Design review of the part built by this model. Coordinates are the model's own, in mm. Face numbers are marked on the shaded views. Round coordinates to 2 decimals unless told otherwise and drop trailing zeros. Loops run counter-clockwise (first coordinate to the right, second up) from the corner with the lowest first, then second, coordinate; pieces in that order, holes last. Notation, with made-up numbers: M 24.5,-4.75 L 69.5,-4.75 A25 cw 69.5,30.25 Z; hole C 74.25,26 d11. An arc over 180 degrees is marked long. One line per item, written item: value. Start each with the question number.
Item 1: We need section C-C (x = 5). Write out the cut boundary in (y, z).
Item 2: We need section D-D (z = 17). Write out the cut boundary in (x, y).
Item 3: Clearance check with flat-ended pins moving along their axes: pin 1 (0.6 mm diameter, centred on y = 4, z = 16, fed in from +X); pin 2 (1.5 mm diameter, centred on x = 3, z = 16, fed in from +Y); pin 3 (1.1 mm diameter, centred on y = 4.5, z = 17, fed in from -X). State where each tip first meets the part, or that it passes through.
Item 4: We need section B-B (z = 5.75). Write out the cut boundary in (x, y), then the cut area to 3 significant figures.
Item 5: For line 1 along Y through (x, z) = (-0.25, 17.25); line 2 along X through (y, z) = (5.5, 25.5); line 3 along X through (y, z) = (-1.75, 7), list the stretches that pass through material, from the lowest coordinate up.
Item 6: Mouldability with a two-part tool opening along X and no side actions: class the marked faces 1, 2 and 3 as released by +X, released by -X, zero draft, split by the parting line, or undercut.
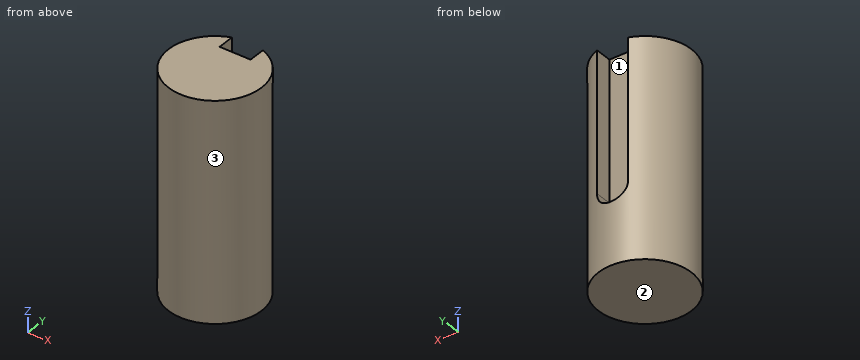
from build123d import *

# Parameters (mm, degrees)
SKETCH1_R           = 6
BOSS_EXTRUDE1_DEPTH = 28
SKETCH2_W           = 4
SKETCH2_H           = 2.5
CUT_EXTRUDE1_DEPTH  = 20
FILLET2_R           = 2
FILLET3_R           = 2


with BuildPart() as part:
    # Sketch1 → Boss-Extrude1 (new body)
    with BuildSketch(Plane.XY):
        Circle(SKETCH1_R)
    extrude(amount=BOSS_EXTRUDE1_DEPTH)

    # Sketch2 → Cut-Extrude1 (cut)
    with BuildSketch(Plane.XY.offset(28)):
        with Locations((0, 4.75)):
            Rectangle(SKETCH2_W, SKETCH2_H)
    extrude(amount=-CUT_EXTRUDE1_DEPTH, mode=Mode.SUBTRACT)

    # Fillet2
    fillet2_edges = [part.edges().sort_by_distance(p)[0] for p in [
        (-2, 4.578427125, 8),
    ]]
    fillet(fillet2_edges, radius=FILLET2_R)

    # Fillet3
    fillet3_edges = [part.edges().sort_by_distance(p)[0] for p in [
        (2, 4.578427125, 8),
    ]]
    fillet(fillet3_edges, radius=FILLET3_R - 0.0001)  # a hair under: the kernel refuses the full size


solid = part.part
A:
1. outline: M -3.32,0 L 3.32,0 L 3.32,28 L -3.32,28 Z
2. outline: M -2,3.5 L -2,5.66 A6 ccw long 2,5.66 L 2,3.5 Z
3. pin 1: x = 4.72
3. pin 2: y = 5.56
3. pin 3: x = -4.52
4. outline: C 0,0 d12
4. area: 113 mm2
5. line 1: -5.99 to 3.5
5. line 2: -2.4 to -2, 2 to 2.4
5. line 3: -5.74 to 5.74
6. face 1: undercut
6. face 2: zero draft
6. face 3: split by the parting line
